Verification items for the finished model (mm, model axes). Face numbers are marked on the shaded views. A direction names the side the tool comes from. Round coordinates to 2 decimals unless told otherwise and drop trailing zeros. Write each loop counter-clockwise with the first axis right and the second up, starting at its lowest first coordinate (ties: lowest second). Pieces come first, ordered by that corner, then holes. Notation, with made-up numbers: (-35.5, 75) - (16.5, 75) arc R21 ccw to (16.5, 112) - close; hole circle Ø4 at (84, 14). An arc over 180 degrees is marked (long way). Answer as a JSON object with one key per item and string values. Group by question number.
1) Section check A-A (y = 0). Enter the section's corners in (x, z) (3 decimals).
2) Section check C-C (z = 6). Enter the section's corners in (x, y).
3) Set-up check for the marked faces 4, 5 and 6: record each of +Z, -Z, +X, -X, +Y, -Y from which the full face is reachable in a straight line by a thin tool's end or side.
4) Go/stop test with flat-tipped pins: pin 1 Ø1.5 at (x, y) = (4, -5.5) entering from +Z; pin 2 Ø5 at (x, y) = (-1, 0) entering from +Z; pin 3 Ø2 at (y, z) = (-10, 29) entering from +X. Record where each tip stops, or that it passes through.
5) Section check D-D (z = 19). Enter the section's corners in (x, y).
6) Thickness scan on line 1 (Y direction, x = 0, z = 35); line 2 (Y direction, x = 8, z = 30.5); line 3 (X direction, y = 4, z = 5.5). Record the ranges inside material, lowest first.
7) Mould release check, pull along Y, two halves, no side actions. Record for the marked faces 1, 2 and 3: +Y half, -Y half, draft (parallel to the pull), parting line (faces both ways), or undercut.
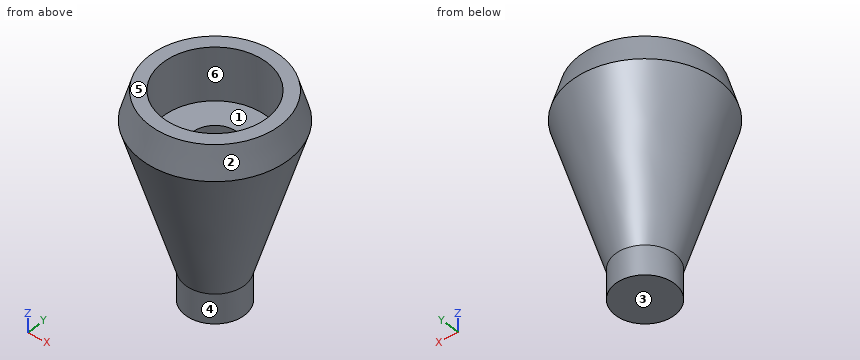
```python
from build123d import *

# Parameters (mm, degrees)
F0_W     = 6.35
F0_H     = 6.35
F2_R     = 11.176
F3_DEPTH = 11.43
F4_R     = 4.826
F5_DEPTH = 38.1


with BuildPart() as f1:
    # F0 (on Front) → F1 (revolve)
    with BuildSketch(Plane.XZ):
        Polygon((0, 38.1), (0, 0), (6.35, 0), (15.875, 31.75), (14.02334, 38.1), align=None)
        with Locations((3.175, -3.175)):
            Rectangle(F0_W, F0_H)
    revolve(axis=Axis((0, 0, 19.05), (0, 0, -1)))

    # F2 (on face) → F3 (cut)
    with BuildSketch(Plane.XY.offset(38.1)):
        Circle(F2_R)
    extrude(amount=-F3_DEPTH, mode=Mode.SUBTRACT)

    # F4 (on face) → F5 (cut)
    with BuildSketch(Plane.XY.offset(38.1)):
        Circle(F4_R)
    extrude(amount=-F5_DEPTH, mode=Mode.SUBTRACT)


solid = f1.part
```
Returned:
{
 "1": {"outline": "(-15.875, 31.75) - (-6.35, 0) - (-6.35, -6.35) - (6.35, -6.35) - (6.35, 0) - (15.875, 31.75) - (14.023, 38.1) - (11.176, 38.1) - (11.176, 26.67) - (4.826, 26.67) - (4.826, 0) - (-4.826, 0) - (-4.826, 26.67) - (-11.176, 26.67) - (-11.176, 38.1) - (-14.023, 38.1) - close"},
 "2": {"outline": "circle Ø16.3 at (0, 0); hole circle Ø9.65 at (0, 0)"},
 "3": {"face 4": "-Z", "face 5": "+Z, +X, -X, +Y, -Y", "face 6": "+Z"},
 "4": {"pin 1": "z = 26.67", "pin 2": "z = 0", "pin 3": "x = 12.15"},
 "5": {"outline": "circle Ø24.1 at (0, 0); hole circle Ø9.65 at (0, 0)"},
 "6": {"line 1": "-14.93 to -11.18, 11.18 to 14.93", "line 2": "-13.28 to -7.8, 7.8 to 13.28", "line 3": "-6.93 to -2.7, 2.7 to 6.93"},
 "7": {"face 1": "undercut", "face 2": "parting line", "face 3": "draft"}
}
